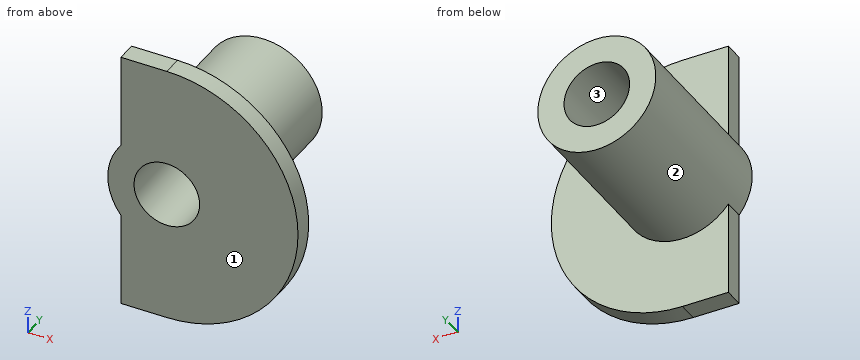
Autodesk Inventor part; units mm, degrees
ref_plane "YZ Plane" through (0, 0, 0) normal (1, 0, 0) x (0, 1, 0)
ref_plane "XZ Plane" through (0, 0, 0) normal (0, 1, 0) x (-1, 0, 0)
ref_plane "XY Plane" through (0, 0, 0) normal (0, 0, 1) x (1, 0, 0)
sketch "Sketch1" plane through (0, 0, 0) normal (0, 1, 0) x (-1, 0, 0)
  circle A0 centre (0, 0) radius 10
  line L0 (0, 10) -> (0, -10)
  line L1 (0, 10) -> (3.5, 10)
  line L2 (3.5, 10) -> (3.5, -10)
  line L3 (3.5, -10) -> (0, -10)
  dimension "d0" = 20
  dimension "d3" = 3.5
extrude "Extrusion1" add sketch "Sketch1" along normal blind 1.5 contours L0 A0 | L1 L2 A0 | A0 L2 L0 | A0 L2 L3
sketch "Sketch3" plane through (0, 1.5, 0) normal (0, 1, 0) x (1, 0, 0)
  circle A0 centre (0, 0) radius 4.5
  circle A1 centre (0, 0) radius 2.5
  dimension "d8" = 9
  dimension "d18" = 5
extrude "Extrusion3" add sketch "Sketch3" along normal blind 10 and the other way blind 1.5
sketch "Sketch4" plane through (0, 11.5, 0) normal (0, 1, 0) x (1, 0, 0)
  line L0 (-3.5, 10) -> (-3.5, 2.8284)
  circle A0 centre (0, 0) radius 4.5
  circle A1 centre (0, 0) radius 2.5
  dimension "d13" = 5
extrude "Extrusion4" add sketch "Sketch4" along normal blind 2 and the other way blind 3
sketch "Sketch2" plane through (0, 1.5, 0) normal (0, 1, 0) x (1, 0, 0)
  circle A0 centre (0, 0) radius 2.5
  circle A1 centre (0, 0) radius 4.5
  dimension "d4" = 5
  dimension "d5" = 9
extrude "Extrusion2" cut sketch "Sketch2" against normal blind 1.5 contours A0
properties part number "Fluorescence_fiber_holder"
Work out the finished part from the listing and answer in its coordinate system (mm). Face numbers are marked on the shaded views. Coordinates: 2 decimals unless noted, no trailing zeros. Write each loop counter-clockwise with the first axis right and the second up, starting at its lowest first coordinate (ties: lowest second). Pieces come first, ordered by that corner, then holes. Notation, with made-up numbers: (4, 20) - (33, 20) arc R23 ccw to (33, 45) - close; hole circle Ø10 at (16, 89.25). An arc over 180 degrees is marked (long way). Answer as a JSON object with one key per item and string values.
Q1. Find section B-B (x = -1.75). Write down the section's boundary in (y, z), plus the area to 3 significant figures.
Results list:
{"outline": "(0, -10) - (1.5, -10) - (1.5, -4.15) - (13.5, -4.15) - (13.5, -1.79) - (0, -1.79) - close; (0, 1.79) - (13.5, 1.79) - (13.5, 4.15) - (1.5, 4.15) - (1.5, 10) - (0, 10) - close", "area": "81.3 mm^2"}
Q2. Given pin 1 Ø3 at (y, z) = (3.5, -3) entering from +X; pin 2 Ø1.5 at (x, z) = (-2, -7) entering from +Y; pin 3 Ø1.6 at (y, z) = (1, 5.5) entering from -X, each flat-ended and moving along its own axis, determine where each tip first touches the part or whether it passes through.
Results list:
{"pin 1": "stops at x = 4.24", "pin 2": "stops at y = 1.5", "pin 3": "stops at x = -3.5"}
Q3. Find section C-C (y = 9.75). Write down the section's boundary in (x, z), plus the area to 3 significant figures.
Results list:
{"outline": "circle Ø9 at (0, 0); hole circle Ø5 at (0, 0)", "area": "44.0 mm^2"}
Q4. Find section A-A (z = 0). Write down the section's boundary in (x, y).
Results list:
{"outline": "(-4.5, 0) - (-2.5, 0) - (-2.5, 13.5) - (-4.5, 13.5) - close; (2.5, 0) - (10, 0) - (10, 1.5) - (4.5, 1.5) - (4.5, 13.5) - (2.5, 13.5) - close"}
Q5. For a pull along Z with two mould halves and no side action, classify the marked faces 1, 2 and 3 as pulls with the +Z half, pulls with the -Z half, needs draft (parallel to the pull), parting line crosses it, or undercut.
Results list:
{"face 1": "needs draft", "face 2": "parting line crosses it", "face 3": "undercut"}
Q6. Consider L1, parallel to X at y = 10.75, z = 0; L2, parallel to Y at x = -2.75, z = 5.75. Determine where each line is inside the solid, lowest interval first. Write a range as from..to.
Results list:
{"L1": "x = -4.5..-2.5, 2.5..4.5", "L2": "y = 0..1.5"}
Q7. Find section D-D (x = 8). Write down the section's boundary in (y, z).
Results list:
{"outline": "(0, -6) - (1.5, -6) - (1.5, 6) - (0, 6) - close"}
